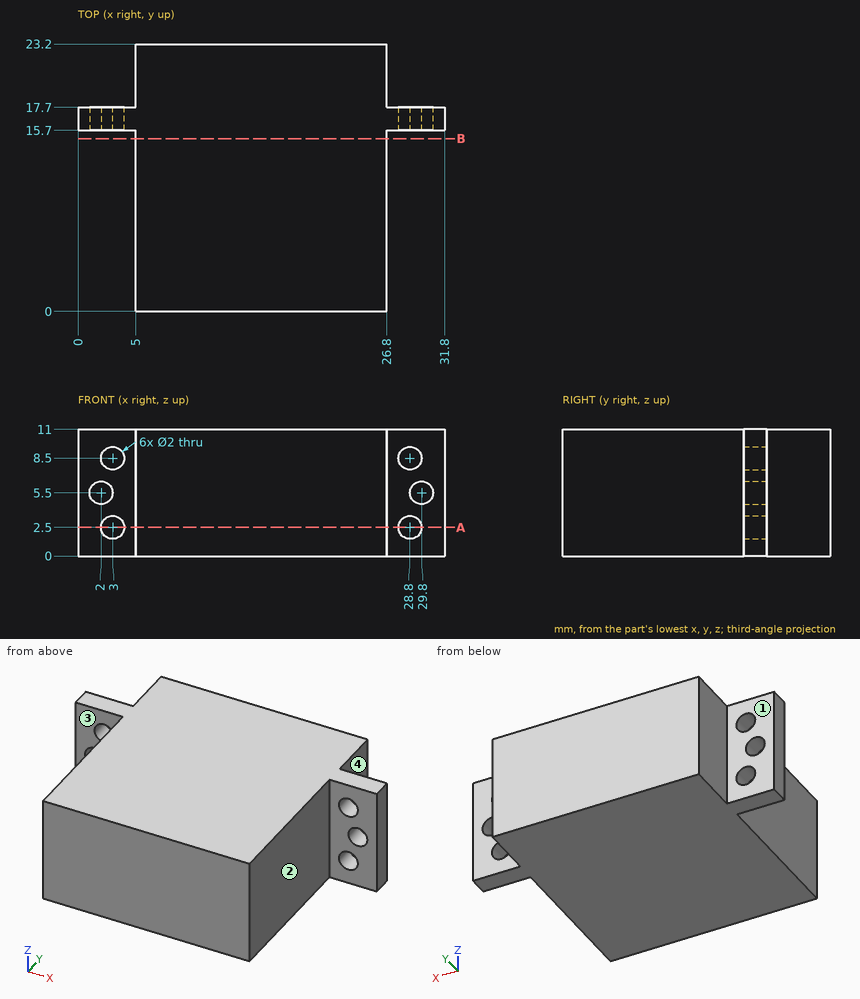
Geometry: see drawing. Coordinates: mm, zero at the bounding-box minimum. A direction names the side the tool comes from. Round coordinates to 2 decimals unless told otherwise and drop trailing zeros. Write each loop counter-clockwise with the first axis right and the second up, starting at its lowest first coordinate (ties: lowest second). Pieces come first, ordered by that corner, then holes. Notation, with made-up numbers: M -10.5,40.25 L -6.5,40.25 A8 cw -6.5,53.25 Z; hole C 29,29.25 d6. An arc over 180 degrees is marked long. Answer in a Markdown table with one row per item. Add a question column.
(1) Cut plane A-A, the plane z = 2.5. Return the cut outline in (x, y), then the cut area to 3 significant figures.
(2) Contact query for flat-ended pins moving along their axis: pin 1 (1.6 mm diameter, centred on y = 20, z = 7, fed in from -X); pin 2 (2.5 mm diameter, centred on x = 3, z = 8.5, fed in from +Y); pin 3 (3 mm diameter, centred on x = 2, z = 5.5, fed in from -Y). Output: stop coordinate, or through.
(3) Reachability of the marked faces 1, 2, 3 and 4 from +Z, -Z, +X, -X, +Y, -Y: full face, straight path, thin tool, end or side. Return the list, or none.
(4) Ray query, L1, parallel to X at y = 13, z = 1.25; L2, parallel to Y at x = 30.5, z = 9.25. Return the intervals inside material, ascending.
(5) Cut plane B-B, the plane y = 15. Return the cut outline in (x, z).
Established:
| question | item | result |
|---|---|---|
| 1 | outline | M 0,15.7 L 2,15.7 L 2,17.7 L 0,17.7 Z; M 4,15.7 L 5,15.7 L 5,0 L 26.8,0 L 26.8,15.7 L 27.8,15.7 L 27.8,17.7 L 26.8,17.7 L 26.8,23.2 L 5,23.2 L 5,17.7 L 4,17.7 Z; M 29.8,15.7 L 31.8,15.7 L 31.8,17.7 L 29.8,17.7 Z |
| 1 | area | 518 mm² |
| 2 | pin 1 | x = 5 |
| 2 | pin 2 | y = 17.7 |
| 2 | pin 3 | y = 15.7 |
| 3 | face 1 | +Z, -Z, -X, +Y |
| 3 | face 2 | +Z, -Z, +X, -Y |
| 3 | face 3 | +Z, -Z, -X, -Y |
| 3 | face 4 | +Z, -Z, +X, +Y |
| 4 | L1 | 5 to 26.8 |
| 4 | L2 | 15.7 to 17.7 |
| 5 | outline | M 5,0 L 26.8,0 L 26.8,11 L 5,11 Z |
